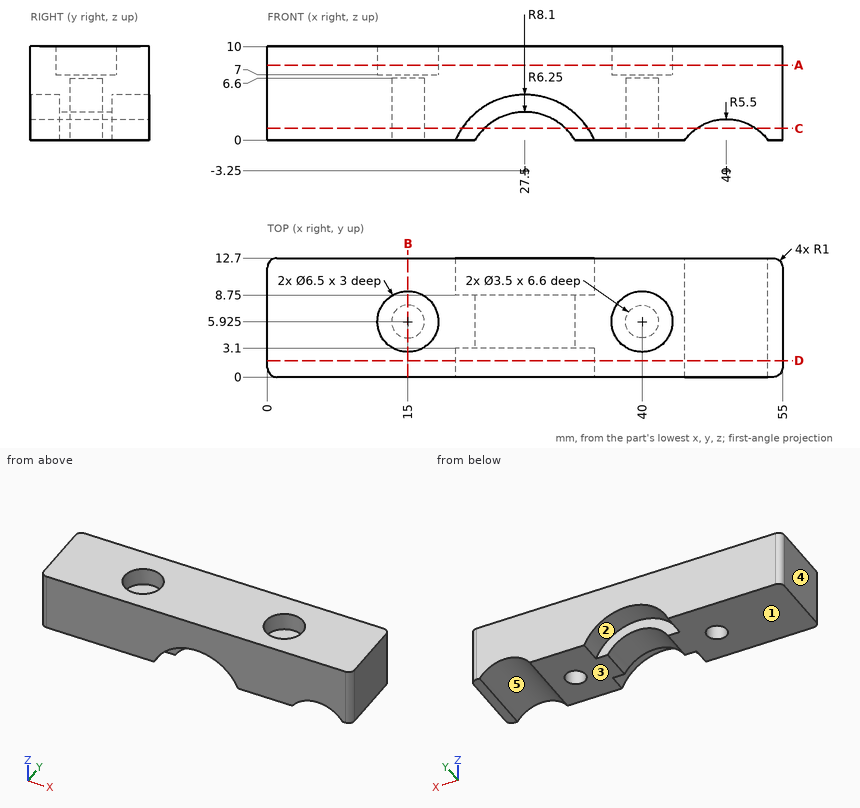
Geometry: see drawing. Coordinates: mm, zero at the bounding-box minimum. A direction names the side the tool comes from. Give positions to 0.01 mm unless a question says otherwise; leave off trailing zeros. Order: outer loops, then holes, each group sorted by start corner. A loop starts at its lowest first (then second) coordinate and runs counter-clockwise, first axis right, second up. Notation, with made-up numbers: (54.5, 28.5) - (59.5, 28.5) arc R13 cw to (59.5, 40.5) - close; hole circle Ø2 at (76, 61). An arc over 180 degrees is marked (long way). One line per item, written item: value.
1. Reachability of the marked faces 1 and 2 from +Z, -Z, +X, -X, +Y, -Y: full face, straight path, thin tool, end or side. Return the list, or none.
Determined:
face 1: -Z, +X, -X, +Y, -Y
face 2: -Z, +Y
2. Line query: probe 1 along Y at (x, z) = (40, 8.45) (3 decimals); probe 2 along X at (y, z) = (7, 9.25); probe 3 along Y at (x, z) = (15, 2) (3 decimals). Output: solid intervals per line, ascending.
Determined:
probe 1: 0 to 2.675, 9.175 to 12.7
probe 2: 0 to 11.93, 18.07 to 36.93, 43.07 to 55
probe 3: 0 to 4.175, 7.675 to 12.7
3. Cut plane B-B, the plane x = 15. Output: boundary loops of the cut face in (y, z) (3 decimals), and give its area (3 significant figures).
Determined:
outline: (0, 0) - (4.175, 0) - (4.175, 6.6) - (7.675, 6.6) - (7.675, 0) - (12.7, 0) - (12.7, 10) - (9.175, 10) - (9.175, 7) - (2.675, 7) - (2.675, 10) - (0, 10) - close
area: 84.4 mm2
4. Cut plane C-C, the plane z = 1.25. Output: boundary loops of the cut face in (x, y) (3 decimals), and give its area (3 significant figures).
Determined:
outline: (0, 1) arc R1 ccw to (1, 0) - (20.765, 0) - (20.765, 3.1) - (23.163, 3.1) - (23.163, 8.75) - (20.765, 8.75) - (20.765, 12.7) - (1, 12.7) arc R1 ccw to (0, 11.7) - close; (31.837, 3.1) - (34.235, 3.1) - (34.235, 0) - (45.838, 0) - (45.838, 12.7) - (34.235, 12.7) - (34.235, 8.75) - (31.837, 8.75) - close; (52.162, 0) - (54, 0) arc R1 ccw to (55, 1) - (55, 11.7) arc R1 ccw to (54, 12.7) - (52.162, 12.7) - close; hole circle Ø3.5 at (15, 5.925); hole circle Ø3.5 at (40, 5.925)
area: 454 mm2
5. Pin query (flat end, axial travel): pin 1 Ø5.5 at (x, y) = (15, 5.925) entering from -Z; pin 2 Ø3 at (x, y) = (40, 5.925) entering from -Z; pin 3 Ø1 at (x, z) = (27.5, 1.5) entering from +Y; pin 4 Ø2.5 at (x, z) = (25.5, 3) entering from -Y. Return the tip coordinate at first contact, or that it passes through.
Determined:
pin 1: z = 0
pin 2: z = 6.6
pin 3: through
pin 4: y = 3.1
6. Cut plane D-D, the plane y = 1.75. Output: boundary loops of the cut face in (x, z).
Determined:
outline: (0, 0) - (20.08, 0) arc R8.1 cw to (34.92, 0) - (44.56, 0) arc R5.5 cw to (53.44, 0) - (55, 0) - (55, 10) - (0, 10) - close
7. Cut plane A-A, the plane z = 8. Output: boundary loops of the cut face in (x, y) (3 decimals), and give its area (3 significant figures).
Determined:
outline: (0, 1) arc R1 ccw to (1, 0) - (54, 0) arc R1 ccw to (55, 1) - (55, 11.7) arc R1 ccw to (54, 12.7) - (1, 12.7) arc R1 ccw to (0, 11.7) - close; hole circle Ø6.5 at (15, 5.925); hole circle Ø6.5 at (40, 5.925)
area: 631 mm2
8. Draft query along X for the marked faces 3, 4 and 5. Return one class per face: released by +X, released by -X, zero draft, split by the parting line, or undercut.
Determined:
face 3: zero draft
face 4: released by -X
face 5: undercut
